Here's how the part is built. I have some questions about the finished solid (model axes, mm). Face numbers are marked on the shaded views. Give positions to 0.01 mm unless a question says otherwise; leave off trailing zeros. Loops run counter-clockwise (first coordinate to the right, second up) from the corner with the lowest first, then second, coordinate; pieces in that order, holes last.
Q1. I'm going to push flat-ended pins straight in: P1, Ø2, axis at x = 15.5, y = 18, coming from the -Z side; P2, Ø10, axis at x = 23, z = 2.5, coming from the +Y side; P3, Ø5.5, axis at x = -10, z = 78.5, coming from the +Y side. Where does each tip first touch, or does it pass through?
Q2. Thinking about a two-plate mould opening in Z: for the marked faces 1, 2 and 3, which applies, pulls with the +Z half, pulls with the -Z half, needs draft (parallel to the pull), parting line crosses it, or undercut?
Q3. Suppose I cut it at A-A (x = 0). List the corners of the cut face in (y, z) for me.
Q4. Suppose I cut it at C-C (y = -2.5). List the corners of the cut face in (x, z) for me.
Q5. I need wall thicknesses on probe 1 along Z at (x, y) = (-2.5, 16); probe 2 along Z at (x, y) = (-67, 10); probe 3 along Y at (x, z) = (13, 77). Which ranges of each line are inside material? Lowest first, please.
Q6. Suppose I cut it at B-B (z = 62.5). List the corners of the cut face in (x, y) for me, and give its area (3 significant figures).
Q7. Suppose I cut it at D-D (x = 30.5). List the corners of the cut face in (y, z) for me, and give its area (4 significant figures).
```python
from build123d import *

# Parameters (mm, degrees)
F0_R     = 19.05
F1_DEPTH = 76.2
F2_W     = 101.6
F2_H     = 38.1
F3_DEPTH = 5
F4_R     = 22.479
F4_R_2   = 19.05
F5_DEPTH = 3
F6_R     = 12.7
F7_DEPTH = 3
F9_DEPTH = 5


with BuildPart() as f1:
    # F0 (on Top) → F1 (new body)
    with BuildSketch(Plane.XY):
        Circle(F0_R)
    extrude(amount=F1_DEPTH)

    # F2 (on face) → F3 (join)
    with BuildSketch(Plane.XY.offset(76.2)):
        with Locations((1.4545911372, -0.3322677247)):
            Rectangle(F2_W, F2_H)
    extrude(amount=F3_DEPTH)

    # F4 (on face) → F5 (join)
    with BuildSketch(Plane(origin=(0, 0, 0), x_dir=(1, 0, 0), z_dir=(0, 0, -1))):
        Circle(F4_R)
        Circle(F4_R_2, mode=Mode.SUBTRACT)
        Circle(F4_R_2)
    extrude(amount=F5_DEPTH)

    # F6 (on face) → F7 (join)
    with BuildSketch(Plane(origin=(0, 0, -3), x_dir=(1, 0, 0), z_dir=(0, 0, -1))):
        Circle(F6_R)
    extrude(amount=F7_DEPTH)

    # F8 (on face) → F9 (join)
    with BuildSketch(Plane.XY.offset(81.2)):
        Polygon((-49.3454088628, -19.3822677247), (-49.3454088628, 18.7177322753), (-148.3056545258, -18.6870153993), align=None)
        Polygon((118.0756762624, -19.3822677247), (52.2545911372, 17.8529117256), (52.2545911372, -19.3822677247), align=None)
    extrude(amount=-F9_DEPTH)


solid = f1.part
```
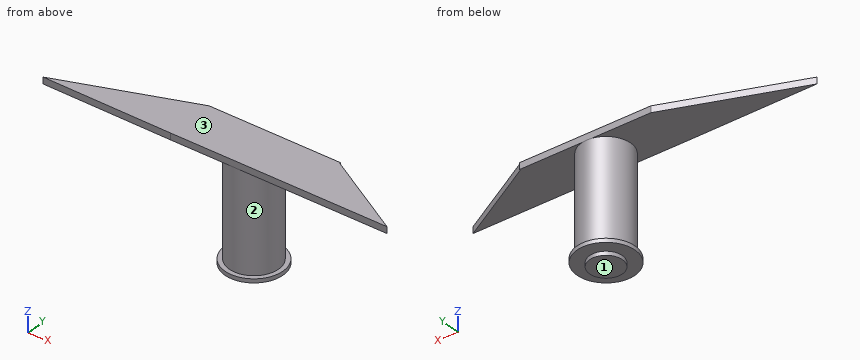
Solutions:
1. P1: stops at z = 76.2
1. P2: stops at y = 12.52
1. P3: stops at y = 18.72
2. face 1: pulls with the -Z half
2. face 2: undercut
2. face 3: pulls with the +Z half
3. outline: (-22.48, -3) - (-12.7, -3) - (-12.7, -6) - (12.7, -6) - (12.7, -3) - (22.48, -3) - (22.48, 0) - (19.05, 0) - (19.05, 76.2) - (18.72, 76.2) - (18.72, 81.2) - (-19.38, 81.2) - (-19.38, 76.2) - (-19.05, 76.2) - (-19.05, 0) - (-22.48, 0) - close
4. outline: (-105.48, 76.2) - (-18.89, 76.2) - (-18.89, 0) - (-22.34, 0) - (-22.34, -3) - (-12.45, -3) - (-12.45, -6) - (12.45, -6) - (12.45, -3) - (22.34, -3) - (22.34, 0) - (18.89, 0) - (18.89, 76.2) - (88.23, 76.2) - (88.23, 81.2) - (-105.48, 81.2) - close
5. probe 1: z = -3 to 81.2
5. probe 2: z = 76.2 to 81.2
5. probe 3: y = -19.38 to 18.72
6. outline: circle Ø38.1 at (0, 0)
6. area: 1,140 mm2
7. outline: (-19.38, 76.2) - (18.72, 76.2) - (18.72, 81.2) - (-19.38, 81.2) - close
7. area: 190.5 mm2
